from build123d import *

# Parameters (mm, degrees)
SKETCH1_R          = 16
SKETCH1_R_2        = 12.5
EXTRUDE1_DEPTH     = 15
SKETCH2_R          = 30
EXTRUDE2_DEPTH     = 6
FILLET1_R          = 2
SKETCH5_W          = 68.7469374
SKETCH5_H          = 68.7469374
CUT_EXTRUDE2_DEPTH = 10


with BuildPart() as part:
    # Sketch1 → Extrude1 (new body)
    with BuildSketch(Plane(origin=(0, 0, 0), x_dir=(1, 0, 0), z_dir=(0, 1, 0))):
        with Locations(Location((0, 0, 0), (0, 0, 270))):
            Circle(SKETCH1_R)
        with Locations(Location((0, 0, 0), (0, 0, 270))):
            Circle(SKETCH1_R_2, mode=Mode.SUBTRACT)
    extrude(amount=EXTRUDE1_DEPTH)

    # Sketch2 → Extrude2 (add)
    with BuildSketch(Plane(origin=(0, 15, 0), x_dir=(1, 0, 0), z_dir=(0, 1, 0))):
        with Locations(Location((0, 0, 0), (0, 0, 270))):
            Circle(SKETCH2_R)
    extrude(amount=EXTRUDE2_DEPTH)

    # Fillet1
    fillet1_edges = [part.edges().sort_by_distance(p)[0] for p in [
        (0, 15, -16),
    ]]
    fillet(fillet1_edges, radius=FILLET1_R)

    # Sketch5 → Cut-Extrude2 (cut)
    with BuildSketch(Plane(origin=(0, 21, 0), x_dir=(1, 0, 0), z_dir=(0, 1, 0))):
        Rectangle(SKETCH5_W, SKETCH5_H)
        Polygon((-21.16926222, 16.16926222), (-16.16926222, 21.16926222), (16.16926222, 21.16926222), (21.16926222, 16.16926222), (21.16926222, -16.16926222), (16.16926222, -21.16926222), (-16.16926222, -21.16926222), (-21.16926222, -16.16926222), align=None, mode=Mode.SUBTRACT)
    extrude(amount=-CUT_EXTRUDE2_DEPTH, mode=Mode.SUBTRACT)


solid = part.part
CAD build for the part. Positions are in the model's coordinates, mm. A direction names the side the tool comes from. Round coordinates to 2 decimals unless told otherwise and drop trailing zeros. Write each loop counter-clockwise with the first axis right and the second up, starting at its lowest first coordinate (ties: lowest second). Pieces come first, ordered by that corner, then holes. Notation, with made-up numbers: M 21.5,67.5 L 57.5,67.5 A25 cw 57.5,82.5 Z; hole C 83.5,-15.75 d3. An arc over 180 degrees is marked long. Use a Markdown table: item, result. Add a question column.
1. Flat gauge pins, fed straight in: P1, Ø1, axis at y = 11.5, z = -8, coming from the +X side; P2, Ø5, axis at x = -8.5, z = 0.5, coming from the -Y side; P3, Ø8, axis at x = -15, y = 3.5, coming from the +Z side. Where does each tip first touch, or does it go through?
2. Slice it at B-B on z = 0. Give the cut face in (x, y).
3. Pull direction Z, two halves, no side cores. Call faces 3 (the face through (21.169, 18, 0)), 4 (the face through (-18.704, 18.042, -18.634)), 5 (the face through (0, 15, 0)), 6 (the face through (3.755, 7.395, 11.923)): released by +Z, released by -Z, zero draft, split by the parting line, or undercut.
4. Slice it at D-D on x = 0. Give the cut face in (y, z), then the cut area to 3 significant figures.
5. Slice it at C-C on y = 11.75. Give the cut face in (x, z).
6. 3-axis set-ups, long thin cutter, end or side, ignore diameter. For faces 1 (the face through (0, 21, 0)), 2 (the face through (-19, 15, 0)): which of +Z, -Z, +X, -X, +Y, -Y reach the whole face in a straight line?
7. Drill centre lines: probe 1 along X at (y, z) = (3.5, 0); probe 2 along Y at (x, z) = (-18, -3.5); probe 3 along X at (y, z) = (14.25, 1). Where is each one in solid material? Low to high.
8. Slice it at A-A on y = 17.25. Give the cut face in (x, z), then the cut area to 3 significant figures.
Reply:
| question | item | result |
|---|---|---|
| 1 | P1 | stops at x = 14.13 |
| 1 | P2 | stops at y = 15 |
| 1 | P3 | stops at z = 11.62 |
| 2 | outline | M -21.17,15 L -18,15 A2 cw -16,13 L -16,0 L -12.5,0 L -12.5,15 L 12.5,15 L 12.5,0 L 16,0 L 16,13 A2 cw 18,15 L 21.17,15 L 21.17,21 L -21.17,21 Z |
| 3 | face 3 | zero draft |
| 3 | face 4 | released by -Z |
| 3 | face 5 | undercut |
| 3 | face 6 | undercut |
| 4 | outline | M 0,-16 L 13,-16 A2 cw 15,-18 L 15,-21.17 L 21,-21.17 L 21,21.17 L 15,21.17 L 15,18 A2 cw 13,16 L 0,16 L 0,12.5 L 15,12.5 L 15,-12.5 L 0,-12.5 Z |
| 4 | area | 361 mm^2 |
| 5 | outline | C 0,0 d32; hole C 0,0 d25 |
| 6 | face 1 | +Z, -Z, +X, -X, +Y |
| 6 | face 2 | -Y |
| 7 | probe 1 | x = -16 to -12.5, 12.5 to 16 |
| 7 | probe 2 | y = 15 to 21 |
| 7 | probe 3 | x = -16.41 to -12.46, 12.46 to 16.41 |
| 8 | outline | M -21.17,-16.17 L -16.17,-21.17 L 16.17,-21.17 L 21.17,-16.17 L 21.17,16.17 L 16.17,21.17 L -16.17,21.17 L -21.17,16.17 Z |
| 8 | area | 1,740 mm^2 |
